Geometry check sheet. Reference: drawing and pictorial views, mm from the part's lowest x, y, z. A direction names the side the tool comes from. Round coordinates to 2 decimals unless told otherwise and drop trailing zeros. Loops run counter-clockwise (first coordinate to the right, second up) from the corner with the lowest first, then second, coordinate; pieces in that order, holes last. Notation, with made-up numbers: (4.25, -30.5) -> (32.25, -30.5) arc R11 ccw to (32.25, -21.5) -> close; hole circle Ø9 at (89, 81). An arc over 180 degrees is marked (long way). Write item = value, one per line.
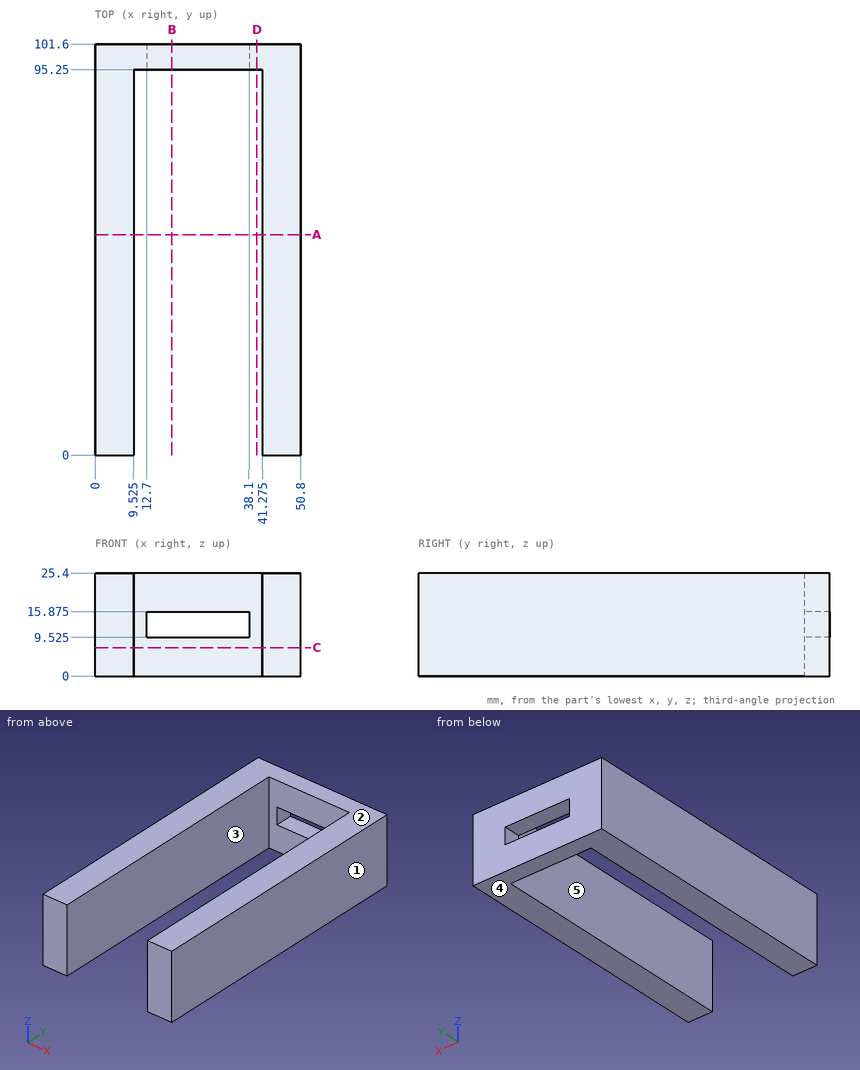
(1) Draft check along X on the marked faces 1, 2 and 3. Enter one of: released by +X, released by -X, zero draft, split by the parting line, or undercut.
Filled sheet:
face_1 = released by +X
face_2 = zero draft
face_3 = undercut
(2) Sectioned sample at B-B, the plane x = 19. Record the cut outline in (y, z) (3 decimals), and give its area (3 significant figures).
Filled sheet:
outline = (95.25, 0) -> (101.6, 0) -> (101.6, 9.525) -> (95.25, 9.525) -> close; (95.25, 15.875) -> (101.6, 15.875) -> (101.6, 25.4) -> (95.25, 25.4) -> close
area = 121 mm2
(3) Set-up check for the marked faces 4 and 5: record each of +Z, -Z, +X, -X, +Y, -Y from which the full face is reachable in a straight line by a thin tool's end or side.
Filled sheet:
face_4 = -Z, +X, -X, +Y, -Y
face_5 = +Z, -Z, -Y
(4) Sectioned sample at C-C, the plane z = 7. Record the cut outline in (x, y) (3 decimals).
Filled sheet:
outline = (0, 0) -> (9.525, 0) -> (9.525, 95.25) -> (41.275, 95.25) -> (41.275, 0) -> (50.8, 0) -> (50.8, 101.6) -> (0, 101.6) -> close
(5) Sectioned sample at D-D, the plane x = 40. Record the cut outline in (y, z).
Filled sheet:
outline = (95.25, 0) -> (101.6, 0) -> (101.6, 25.4) -> (95.25, 25.4) -> close
(6) Sectioned sample at A-A, the plane y = 54.5. Record the cut outline in (x, z) (3 decimals), and give its area (3 significant figures).
Filled sheet:
outline = (0, 0) -> (9.525, 0) -> (9.525, 25.4) -> (0, 25.4) -> close; (41.275, 0) -> (50.8, 0) -> (50.8, 25.4) -> (41.275, 25.4) -> close
area = 484 mm2
(7) Material ranges on probe 1 along X at (y, z) = (42, 9.25) (3 decimals); probe 2 along Y at (x, z) = (30.5, 23), recorded low to high. Write a range as from..to.
Filled sheet:
probe_1 = 0..9.525, 41.275..50.8
probe_2 = 95.25..101.6
(8) Go/stop test with a flat-tipped pin: pin 1 Ø1 at (x, z) = (28.5, 10.5) entering from -Y. Record where the tip stops, or that it passes through.
Filled sheet:
pin_1 = through
